Source: CAD feature listing. Evaluate the final solid. Frame: model axes, mm. A direction names the side the tool comes from. Round coordinates to 2 decimals unless told otherwise and drop trailing zeros. Write each loop counter-clockwise with the first axis right and the second up, starting at its lowest first coordinate (ties: lowest second). Pieces come first, ordered by that corner, then holes. Notation, with made-up numbers: (88, -34.5) - (109, -34.5) arc R15 ccw to (109, -29.5) - close; hole circle Ø1 at (78.25, 86.25). An arc over 180 degrees is marked (long way). Write item = value, one per line. Start each with the question number.
```python
from build123d import *

# Parameters (mm, degrees)
SKETCH1_W            = 83
SKETCH1_H            = 83
BOSS_EXTRUDE1_DEPTH  = 6
SKETCH2_R            = 1
CUT_EXTRUDE1_DEPTH   = 6
LPATTERN1_COUNT      = 2
LPATTERN1_PITCH      = 72
LPATTERN1_COUNT_DIR2 = 2
LPATTERN1_PITCH_DIR2 = 60
SKETCH3_R            = 1
CUT_EXTRUDE2_DEPTH   = 10


with BuildPart() as part:
    # Sketch1 → Boss-Extrude1 (new body)
    with BuildSketch(Plane(origin=(0, 0, 0), x_dir=(1, 0, 0), z_dir=(0, 1, 0))):
        with Locations((41.5, 41.5)):
            Rectangle(SKETCH1_W, SKETCH1_H)
    extrude(amount=BOSS_EXTRUDE1_DEPTH)

    # Sketch2 → Cut-Extrude1 (cut)
    with BuildSketch(Plane(origin=(0, 6, 0), x_dir=(1, 0, 0), z_dir=(0, 1, 0))):
        with Locations(Location((6, 71, 0), (0, 0, 270))):
            Circle(SKETCH2_R)
    cut_extrude1 = extrude(amount=-CUT_EXTRUDE1_DEPTH, mode=Mode.SUBTRACT)

    # LPattern1: Cut-Extrude1 2 × 2
    with Locations(*[(i * LPATTERN1_PITCH, 0, j * LPATTERN1_PITCH_DIR2) for i in range(LPATTERN1_COUNT) for j in range(LPATTERN1_COUNT_DIR2) if (i, j) != (0, 0)]):
        add(cut_extrude1, mode=Mode.SUBTRACT)

    # Sketch3 → Cut-Extrude2 (cut)
    with BuildSketch(Plane.ZY):
        with Locations((-78, 3)):
            Circle(SKETCH3_R)
        with Locations((-5, 3)):
            Circle(SKETCH3_R)
    cut_extrude2 = extrude(amount=-CUT_EXTRUDE2_DEPTH, mode=Mode.SUBTRACT)

    # Mirror1: Cut-Extrude2 across plane
    add(cut_extrude2.mirror(Plane.ZY.offset(-41.5)), mode=Mode.SUBTRACT)


solid = part.part
```
(1) Contact query for flat-ended pins moving along their axis: P1, Ø1.8, axis at y = 3, z = -5, coming from the +X side; P2, Ø1.6, axis at x = 78, z = -11, coming from the +Y side; P3, Ø1.2, axis at y = 3, z = -78, coming from the -X side. Output: stop coordinate, or through.
(2) Ray query, L1, parallel to X at y = 2.7, z = -71; L2, parallel to Y at x = 75, z = -78; L3, parallel to Z at x = 79.5, y = 2.1. Return the intervals inside material, ascending. Write a range as from..to.
(3) Pull-direction query (Y, two-part tool) for faces 1 (the cylindrical face through (7, 3, -11)), 2 (the cylindrical face through (78.07, 3.676, -5.737)), 3 (the flat face through (41, 6, -42)); classes: +Y half, -Y half, draft (parallel to the pull), parting line (faces both ways), or undercut.
(4) Section B-B (x = 78). Return the cut outline in (y, z).
(5) Section A-A (z = -11). Return the cut outline in (x, y).
(6) Reachability of faces 4 (the flat face through (73, 3, -78)), 5 (the flat face through (41, 3, 0)), 6 (the cylindrical face through (4.93, 3.676, -5.737)) from +Z, -Z, +X, -X, +Y, -Y: full face, straight path, thin tool, end or side. Return the list, or none.
(7) Section C-C (z = -78). Return the cut outline in (x, y).
Solution:
q1.P1 = 73
q1.P2 = through
q1.P3 = 10
q2.L1 = 0..5, 7..77, 79..83
q2.L2 = 0..2, 4..6
q2.L3 = -83..-78.44, -77.56..-5.44, -4.56..0
q3.face_1 = draft
q3.face_2 = undercut
q3.face_3 = +Y half
q4.outline = (0, -83) - (6, -83) - (6, -72) - (0, -72) - close; (0, -70) - (6, -70) - (6, -12) - (0, -12) - close; (0, -10) - (6, -10) - (6, 0) - (0, 0) - close; hole circle Ø2 at (3, -78); hole circle Ø2 at (3, -5)
q5.outline = (0, 0) - (5, 0) - (5, 6) - (0, 6) - close; (7, 0) - (77, 0) - (77, 6) - (7, 6) - close; (79, 0) - (83, 0) - (83, 6) - (79, 6) - close
q6.face_4 = +X
q6.face_5 = +Z, +X, -X, +Y, -Y
q6.face_6 = -X
q7.outline = (0, 0) - (83, 0) - (83, 2) - (73, 2) - (73, 4) - (83, 4) - (83, 6) - (0, 6) - (0, 4) - (10, 4) - (10, 2) - (0, 2) - close
